Autodesk Inventor part; units mm, degrees
ref_plane "YZ Plane" through (0, 0, 0) normal (1, 0, 0) x (0, 1, 0)
ref_plane "XZ Plane" through (0, 0, 0) normal (0, 1, 0) x (-1, 0, 0)
ref_plane "XY Plane" through (0, 0, 0) normal (0, 0, 1) x (1, 0, 0)
sketch "Sketch1" plane through (0, 0, 0) normal (0, 0, 1) x (1, 0, 0)
  line L0 (0, 0) -> (14.5, 0)
  line L1 (14.5, 0) -> (14.5, 6.8)
  line L2 (14.5, 6.8) -> (0, 6.8)
  line L3 (0, 6.8) -> (0, 0)
  dimension "d0" = 14.5
  dimension "d1" = 6.8
extrude "Extrusion1" add sketch "Sketch1" along normal blind 1.6
sketch "Sketch2" plane through (0, 0, 1.6) normal (0, 0, 1) x (1, 0, 0)
  line L0 (0, 6.8) -> (0, 0)
  line L1 (0, 6.8) -> (2.5, 6.8)
  line L2 (2.5, 6.8) -> (2.5, 5.2)
  line L3 (2.5, 5.2) -> (0, 5.2)
  line L4 (0, 5.2) -> (0, 6.8)
  line L5 (0, 0) -> (2.5, 0)
  line L6 (2.5, 0) -> (2.5, 1.6)
  line L7 (2.5, 1.6) -> (0, 1.6)
  line L8 (0, 1.6) -> (0, 0)
  line L9 (0, 0) -> (14.5, 0)
  line L10 (14.5, 0) -> (12, 0)
  line L11 (12, 0) -> (12, 1.6)
  line L12 (12, 1.6) -> (14.5, 1.6)
  line L13 (14.5, 1.6) -> (14.5, 0)
  line L14 (14.5, 0) -> (14.5, 6.8)
  line L15 (14.5, 6.8) -> (12, 6.8)
  line L16 (12, 6.8) -> (12, 5.2)
  line L17 (12, 5.2) -> (14.5, 5.2)
  line L18 (14.5, 5.2) -> (14.5, 6.8)
  dimension "d4" = 2.5
  dimension "d5" = 1.6
  dimension "d6" = 2.5
  dimension "d7" = 1.6
  dimension "d8" = 2.5
  dimension "d9" = 1.6
  dimension "d10" = 1.6
extrude "Extrusion2" add sketch "Sketch2" along normal blind 10
properties part number "ButtonLock"
Can you work these out from the model? Positions are in its coordinate system, mm. A direction names the side the tool comes from. Round coordinates to 2 decimals unless told otherwise and drop trailing zeros. Order: outer loops, then holes, each group sorted by start corner. A loop starts at its lowest first (then second) coordinate and runs counter-clockwise, first axis right, second up. Notation, with made-up numbers: (-25.75, -5) - (-19.75, -5) arc R24 cw to (-19.75, 33) - close; hole circle Ø8 at (57.25, -24.75). An arc over 180 degrees is marked (long way). Answer in a Markdown table with one row per item.
(1) Suppose I cut it at D-D, the plane y = 4. Please give me the cut outline in (x, z), plus the area to 3 significant figures.
From the geometry:
| item | result |
|---|---|
| outline | (0, 0) - (14.5, 0) - (14.5, 1.6) - (0, 1.6) - close |
| area | 23.2 mm2 |
(2) Please list where these lines run through material, in increasing order: L1, parallel to X at y = 5.5, z = 2.5; L2, parallel to Y at x = 13.5, z = 11.25; L3, parallel to Z at x = 9.5, y = 1.75. Write a range as from..to.
From the geometry:
| item | result |
|---|---|
| L1 | x = 0..2.5, 12..14.5 |
| L2 | y = 0..1.6, 5.2..6.8 |
| L3 | z = 0..1.6 |
(3) Which directions (+Z, -Z, +X, -X, +Y, -Y) give clear straight access to the entire face, cutting with the end or side of a thin tool? Please do faces 5 (the face through (13, 5.2, 7)), 6 (the face through (13, 1, 11.6)), 7 (the face through (2.5, 6, 7)).
From the geometry:
| item | result |
|---|---|
| face 5 | +Z, +X, -X |
| face 6 | +Z, +X, -X, +Y, -Y |
| face 7 | +Z, +Y, -Y |
(4) If we mould it in two halves opening along X, with no side actions, what happens to faces 1 (the face through (2.5, 1, 7)), 2 (the face through (12, 6, 7)), 3 (the face through (14.5, 6, 6)), 4 (the face through (12.2, 6.8, 4.4))? For each: released by +X, released by -X, zero draft, split by the parting line, or undercut.
From the geometry:
| item | result |
|---|---|
| face 1 | undercut |
| face 2 | undercut |
| face 3 | released by +X |
| face 4 | zero draft |
(5) Suppose I cut it at C-C, the plane y = 5.75. Please give me the cut outline in (x, z).
From the geometry:
| item | result |
|---|---|
| outline | (0, 0) - (14.5, 0) - (14.5, 11.6) - (12, 11.6) - (12, 1.6) - (2.5, 1.6) - (2.5, 11.6) - (0, 11.6) - close |
(6) For P1, Ø1.8, axis at y = 6, z = 7.5, coming from the -X side; P2, Ø1.5, axis at x = 4, y = 6, coming from the +Z side, each with a flat end and sliding along its axis, tell me the tip position at first contact or that it passes through.
From the geometry:
| item | result |
|---|---|
| P1 | stops at x = 0 |
| P2 | stops at z = 1.6 |
(7) Suppose I cut it at A-A, the plane z = 10.25. Please give me the cut outline in (x, y).
From the geometry:
| item | result |
|---|---|
| outline | (0, 0) - (2.5, 0) - (2.5, 1.6) - (0, 1.6) - close; (0, 5.2) - (2.5, 5.2) - (2.5, 6.8) - (0, 6.8) - close; (12, 0) - (14.5, 0) - (14.5, 1.6) - (12, 1.6) - close; (12, 5.2) - (14.5, 5.2) - (14.5, 6.8) - (12, 6.8) - close |
(8) Suppose I cut it at B-B, the plane x = 1.5. Please give me the cut outline in (y, z).
From the geometry:
| item | result |
|---|---|
| outline | (0, 0) - (6.8, 0) - (6.8, 11.6) - (5.2, 11.6) - (5.2, 1.6) - (1.6, 1.6) - (1.6, 11.6) - (0, 11.6) - close |
